```python
from build123d import *

# Parameters (mm, degrees)
HV_TOP_PANEL_DEPTH                   = 107.95
SKETCH10_W                           = 73.025
SKETCH10_H                           = 415.925
INTERFACE_WITH_BACK_COVER_DEPTH      = 78.74
SKETCH11_W                           = 334.01
SKETCH11_H                           = 19.05
INTEFACE_WITH_MOTOR_DISCONNECT_DEPTH = 74.93
CUT_EXTRUDE6_DEPTH                   = 87.63
SKETCH14_W                           = 10.16
SKETCH14_H                           = 239.7125
CUT_EXTRUDE3_DEPTH                   = 29.21
SHELL1_T                             = 3.175
SKETCH17_W                           = 39.6875
SKETCH17_H                           = 3.175
SKETCH17_W_2                         = 23.8125
OVERLAP_ON_LID_DEPTH                 = 12.7
LIP_DEPTH                            = 19.05
SKETCH18_W                           = 49.2125
SKETCH18_H                           = 209.55
MOTOR_DISCONNECT_DEPTH               = 7.62
SKETCH19_W                           = 44.45
SKETCH19_H                           = 105.664
SKETCH19_W_2                         = 171.45
SKETCH19_H_2                         = 79.375
LV_AND_HV_PANELS_DEPTH               = 7.62


with BuildPart() as part:
    # Sketch4 → HV Top Panel (new body)
    with BuildSketch(Plane(origin=(0, 0, 0), x_dir=(1, 0, 0), z_dir=(0, 1, 0))):
        Polygon((176.607773845, -221.387726412), (-167.562226155, -221.387726412), (-167.562226155, -219.800226412), (-167.562226155, 131.037273588), (176.607773845, 131.037273588), align=None)
    extrude(amount=HV_TOP_PANEL_DEPTH)

    # Sketch10 → Interface with Back Cover (add)
    with BuildSketch(Plane(origin=(0, 0, 0), x_dir=(1, 0, 0), z_dir=(0, 1, 0))):
        with Locations((213.120273845, -37.237726412)):
            Rectangle(SKETCH10_W, SKETCH10_H)
    extrude(amount=INTERFACE_WITH_BACK_COVER_DEPTH)

    # Sketch11 → Inteface with Motor Disconnect (cut)
    with BuildSketch(Plane(origin=(0, 107.95, 0), x_dir=(1, 0, 0), z_dir=(0, 1, 0))):
        with Locations((-0.557226155, -211.862726412)):
            Rectangle(SKETCH11_W, SKETCH11_H)
    extrude(amount=-INTEFACE_WITH_MOTOR_DISCONNECT_DEPTH, mode=Mode.SUBTRACT)

    # Sketch11<3> → Cut-Extrude6 (cut)
    with BuildSketch(Plane(origin=(0, 107.95, 0), x_dir=(1, 0, 0), z_dir=(0, 1, 0))):
        Polygon((166.447773845, -245.200226412), (249.632773845, -245.200226412), (249.632773845, -169.000226412), (176.607773845, -169.000226412), (176.607773845, -221.387726412), (166.447773845, -221.387726412), align=None)
        Polygon((166.447773845, -202.337726412), (166.447773845, -221.387726412), (176.607773845, -221.387726412), (176.607773845, -169.000226412), (166.447773845, -169.000226412), align=None)
        Polygon((176.607773845, 131.037273588), (176.607773845, 97.699773588), (249.632773845, 97.699773588), (249.632773845, 170.724773588), (176.607773845, 170.724773588), align=None)
    extrude(amount=-CUT_EXTRUDE6_DEPTH, mode=Mode.SUBTRACT)

    # Sketch14 → Cut-Extrude3 (cut)
    with BuildSketch(Plane(origin=(0, 107.95, 0), x_dir=(1, 0, 0), z_dir=(0, 1, 0))):
        with Locations((171.527773845, -49.143976412)):
            Rectangle(SKETCH14_W, SKETCH14_H)
    extrude(amount=-CUT_EXTRUDE3_DEPTH, mode=Mode.SUBTRACT)

    # Shell1
    shell1_openings = [part.faces().sort_by_distance(p)[0] for p in [
        (46.296622828, 0, 43.585658338),
    ]]
    offset(amount=SHELL1_T, openings=shell1_openings, kind=Kind.INTERSECTION)

    # Sketch17 → Overlap on Lid (add)
    with BuildSketch(Plane.ZY.offset(-173.432773845)):
        with Locations((-154.056023588, 1.5875)):
            Rectangle(SKETCH17_W, SKETCH17_H)
        with Locations((236.468976412, 1.5875)):
            Rectangle(SKETCH17_W_2, SKETCH17_H)
    extrude(amount=OVERLAP_ON_LID_DEPTH)

    # Sketch15 → Lip (add)
    with BuildSketch(Plane.XZ):
        Polygon((249.632773845, 245.200226412), (249.632773845, -170.724773588), (176.607773845, -170.724773588), (160.732773845, -170.724773588), (160.732773845, -173.899773588), (252.807773845, -173.899773588), (252.807773845, 248.375226412), (160.732773845, 248.375226412), (160.732773845, 245.200226412), (176.607773845, 245.200226412), align=None)
    extrude(amount=LIP_DEPTH)

    # Sketch18 → Motor Disconnect (cut)
    with BuildSketch(Plane(origin=(0, 81.915, 0), x_dir=(1, 0, 0), z_dir=(0, 1, 0))):
        with Locations((202.166523845, -37.237726412)):
            Rectangle(SKETCH18_W, SKETCH18_H)
    extrude(amount=-MOTOR_DISCONNECT_DEPTH, mode=Mode.SUBTRACT)

    # Sketch19 → LV and HV Panels (cut)
    with BuildSketch(Plane(origin=(0, 0, -134.212273588), x_dir=(-1, 0, 0), z_dir=(0, 0, -1))):
        with Locations((-151.207773845, 52.832)):
            Rectangle(SKETCH19_W, SKETCH19_H)
        with Locations((81.837226155, 39.6875)):
            Rectangle(SKETCH19_W_2, SKETCH19_H_2)
    extrude(amount=-LV_AND_HV_PANELS_DEPTH, mode=Mode.SUBTRACT)


solid = part.part
```
Verification items for the finished model (mm, model axes). A direction names the side the tool comes from. Coordinates: 2 decimals unless noted, no trailing zeros. Loops run counter-clockwise (first coordinate to the right, second up) from the corner with the lowest first, then second, coordinate; pieces in that order, holes last. Notation, with made-up numbers: (71, 88.5) - (97, 88.5) arc R12 ccw to (97, 107.5) - close; hole circle Ø11 at (-30.75, -37). An arc over 180 degrees is marked (long way). Return JSON: item names as keys, results as strings.
1. Section check A-A, the plane z = -9.5. Record the boundary of the cut face in (x, y) (3 decimals), then the cut area to 3 significant figures.
Established:
{"outline": "(-170.737, 0) - (-167.562, 0) - (-167.562, 107.95) - (166.448, 107.95) - (166.448, 78.74) - (177.56, 78.74) - (177.56, 81.915) - (169.623, 81.915) - (169.623, 111.125) - (-170.737, 111.125) - close; (226.773, 78.74) - (249.633, 78.74) - (249.633, -19.05) - (252.808, -19.05) - (252.808, 81.915) - (226.773, 81.915) - close", "area": "1,930 mm2"}
2. Section check B-B, the plane y = 45. Record the boundary of the cut face in (x, z), then the cut area to 3 significant figures.
Established:
{"outline": "(-170.74, -134.21) - (-167.56, -134.21) - (-167.56, 202.34) - (166.45, 202.34) - (166.45, 169) - (249.63, 169) - (249.63, -97.7) - (176.61, -97.7) - (176.61, -131.04) - (173.43, -131.04) - (173.43, -134.21) - (179.78, -134.21) - (179.78, -100.87) - (252.81, -100.87) - (252.81, 172.18) - (169.62, 172.18) - (169.62, 205.51) - (-170.74, 205.51) - close; (3.89, -134.21) - (128.98, -134.21) - (128.98, -131.04) - (3.89, -131.04) - close", "area": "4,120 mm2"}
3. Section check D-D, the plane z = -140.5. Record the boundary of the cut face in (x, y) (3 decimals), then the cut area to 3 significant figures.
Established:
{"outline": "(160.733, 0) - (176.608, 0) - (176.608, 20.32) - (249.633, 20.32) - (249.633, -19.05) - (252.808, -19.05) - (252.808, 23.495) - (173.433, 23.495) - (173.433, 3.175) - (160.733, 3.175) - close", "area": "482 mm2"}
4. Thickness scan on L1, parallel to X at y = 84, z = -79; L2, parallel to X at y = 96, z = -24; L3, parallel to Z at x = 226.5, y = 66. Record the ranges inside material, lowest first.
Established:
{"L1": "x = -170.74 to -167.56, 176.61 to 179.78", "L2": "x = -170.74 to -167.56, 166.45 to 169.62", "L3": "z = -100.87 to -97.7, 169 to 172.18"}
5. Go/stop test with flat-tipped pins: pin 1 (3.5 mm diameter, centred on y = 34.5, z = -132.5, fed in from +X); pin 2 (1 mm diameter, centred on x = 4.5, z = -32, fed in from -Y); pin 3 (1.6 mm diameter, centred on x = -61.5, z = -132.5, fed in from -Y) (3 decimals). Record where each tip stops, or that it passes through.
Established:
{"pin 1": "stops at x = 179.78", "pin 2": "stops at y = 107.95", "pin 3": "stops at y = 79.375"}
6. Section check C-C, the plane x = -18. Record the boundary of the cut face in (y, z) (3 decimals), then the cut area to 3 significant figures.
Established:
{"outline": "(0, 221.388) - (33.02, 221.388) - (33.02, 202.338) - (107.95, 202.338) - (107.95, -131.037) - (79.375, -131.037) - (79.375, -134.212) - (111.125, -134.212) - (111.125, 205.513) - (36.195, 205.513) - (36.195, 224.563) - (0, 224.563) - close", "area": "1,570 mm2"}
7. Tool access check on faces 4 (the flat face through (160.733, 0.3, 241.8)), 5 (the flat face through (173.433, 13, 237)), 6 (the flat face through (-167.562, 53, 41)), 7 (the flat face through (211, 23.495, 210)), 8 (the flat face through (167, 3.175, -154)). Record the directions out of +Z, -Z, +X, -X, +Y, -Y that give a thin tool (end or side, any length) a straight path to the whole face; none if there is none.
Established:
{"face 4": "+Z, -X, +Y, -Y", "face 5": "+Z, -X, +Y", "face 6": "-Y", "face 7": "+Z, +X, +Y", "face 8": "-Z, -X, +Y"}
8. Mould release check, pull along Z, two halves, no side actions. Record for faces 1 (the flat face through (-3, 33.02, 212)), 2 (the flat face through (207, 3, 248.375)), 3 (the flat face through (-3, 36.195, 215)): +Z half, -Z half, draft (parallel to the pull), parting line (faces both ways), or undercut.
Established:
{"face 1": "undercut", "face 2": "+Z half", "face 3": "draft"}
